from build123d import *

# Parameters (mm, degrees)
CHAMFER_1_SIZE = 1
SKETCH_4_W     = 3
SKETCH_4_H     = 3
FILLET_1_R     = 1
CHAMFER_2_SIZE = 0.4


with BuildPart() as part:
    # 草图3 → 旋转1 (revolve)
    with BuildSketch(Plane.XY, mode=Mode.PRIVATE) as revolve_1_sk:
        Polygon((0, 0), (0, 14.035898385), (6, 17.5), (70, 17.5), (70, 9), (100, 9), (100, 0), align=None)
    revolve(revolve_1_sk.sketch.rotate(Axis((100, 0, 0), (-1, 0, 0)), 90), axis=Axis((100, 0, 0), (-1, 0, 0)))

    # 倒角1
    chamfer_1_edges = [part.edges().sort_by_distance(p)[0] for p in [
        (100, 0, 9),
    ]]
    chamfer(chamfer_1_edges, length=CHAMFER_1_SIZE)

    # 草图4 → 切除-旋转1 (revolve, cut)
    with BuildSketch(Plane.XY, mode=Mode.PRIVATE) as cut_revolve_1_sk:
        with Locations((71.1, 10.1)):
            Rectangle(SKETCH_4_W, SKETCH_4_H)
    revolve(cut_revolve_1_sk.sketch.rotate(Axis((66.500454026, 0, 0), (1, 0, 0)), 90), axis=Axis((66.500454026, 0, 0), (1, 0, 0)), mode=Mode.SUBTRACT)

    # 圆角1
    fillet_1_edges = [part.edges().sort_by_distance(p)[0] for p in [
        (69.6, 0, -8.6),
    ]]
    fillet(fillet_1_edges, radius=FILLET_1_R)

    # 倒角2
    chamfer_2_edges = [part.edges().sort_by_distance(p)[0] for p in [
        (72.6, 0, -8.6),
        (69.6, 0, -11.6),
    ]]
    chamfer(chamfer_2_edges, length=CHAMFER_2_SIZE - 0.0001)  # a hair under: the kernel refuses the full size


solid = part.part
The model under review builds one solid part; all positions refer to its coordinate system, in mm. A direction names the side the tool comes from. Round coordinates to 2 decimals unless told otherwise and drop trailing zeros. Order: outer loops, then holes, each group sorted by start corner. A loop starts at its lowest first (then second) coordinate and runs counter-clockwise, first axis right, second up. Notation, with made-up numbers: (62.25, 48) -> (117.25, 48) arc R11 cw to (117.25, 61) -> close; hole circle Ø4 at (37, 55). An arc over 180 degrees is marked (long way). Return JSON: item names as keys, results as strings.
1. For L1, parallel to X at y = -9.5, z = 7; L2, parallel to X at y = -4.5, z = 8.5; L3, parallel to Y at x = 22.5, z = -1, list the stretches that pass through material, from the lowest coordinate up. Write a range as [from, to].
Answer block:
{"L1": "x = [0, 70]", "L2": "x = [0, 69.6]", "L3": "y = [-17.47, 17.47]"}
2. Take a section at C-C (x = 11). Write out the cut boundary in (y, z).
Answer block:
{"outline": "circle Ø35 at (0, 0)"}
3. Take a section at D-D (x = 92.5). Write out the cut boundary in (y, z), then the cut area to 3 significant figures.
Answer block:
{"outline": "circle Ø18 at (0, 0)", "area": "254 mm²"}
4. Insertion check: P1, Ø12, axis at x = 13.5, z = 10, coming from the +Y side; P2, Ø12, axis at x = 36.5, z = 8.5, coming from the +Y side; P3, Ø4, axis at x = 85.5, y = 3.5, coming from the -Z side. Each pin has a flat end and moves straight along its axis. Give the tip position at first contact, or say it passes through.
Answer block:
{"P1": "stops at y = 17.04", "P2": "stops at y = 17.32", "P3": "stops at z = -8.87"}
5. For faces 1 (the face through (70, 11.4, -3.6)), 2 (the face through (38.448, 17.084, 3.794)), list the 3-axis set-ups (+Z, -Z, +X, -X, +Y, -Y) from which the entire face can be reached by the end or side of a thin tool; tool diameter is ignored.
Answer block:
{"face 1": "+X", "face 2": "+X, -X"}
6. The part is to be moulded in two halves that separate along Z. For faces 3 (the face through (0, 0, 0)), 4 (the face through (71.41, -0.38, -8.59)), say which applies: +Z half, -Z half, draft (parallel to the pull), parting line (faces both ways), or undercut.
Answer block:
{"face 3": "draft", "face 4": "parting line"}
